Input: part model. Units: mm. Frame: model coordinates. A direction names the side the tool comes from. Give positions to 0.01 mm unless a question says otherwise; leave off trailing zeros. Loops run counter-clockwise (first coordinate to the right, second up) from the corner with the lowest first, then second, coordinate; pieces in that order, holes last. Notation, with made-up numbers: (35.25, 72) -> (80.25, 72) arc R23 cw to (80.25, 95) -> close; hole circle Ø6 at (-6, 24). An arc over 180 degrees is marked (long way). Answer as a JSON object with one key per item and string values. Group by question number.
```python
from build123d import *

# Parameters (mm, degrees)
SKETCH1_R                  = 9
SKETCH1_R_2                = 6
MAIN_DEPTH                 = 9.5
SKETCH2_W                  = 25
SKETCH2_H                  = 19
SKETCH2_R                  = 4
SKETCH2_R_2                = 1.35
BALLSUPPORTEXTRUSION_DEPTH = 5
SKETCH3_R                  = 5.15
BALLSUPPORTHOLE_DEPTH      = 4
FILLET2_R                  = 2
SKETCH5_R                  = 6
CUT_EXTRUDE2_DEPTH         = 20


with BuildPart() as part:
    # Sketch1 → Main (new body, symmetric)
    with BuildSketch(Plane.XY):
        Circle(SKETCH1_R)
        Circle(SKETCH1_R_2, mode=Mode.SUBTRACT)
    extrude(amount=MAIN_DEPTH, both=True)

    # Sketch2 → BallSupportExtrusion (add)
    with BuildSketch(Plane(origin=(0, -9, 0), x_dir=(1, 0, 0), z_dir=(0, 1, 0))):
        with Locations((12.5, 0)):
            Rectangle(SKETCH2_W, SKETCH2_H)
        with Locations((18, 0)):
            Circle(SKETCH2_R, mode=Mode.SUBTRACT)
        with Locations((18, 7)):
            Circle(SKETCH2_R_2, mode=Mode.SUBTRACT)
        with Locations((18, -7)):
            Circle(SKETCH2_R_2, mode=Mode.SUBTRACT)
    extrude(amount=BALLSUPPORTEXTRUSION_DEPTH)

    # Sketch3 → BallSupportHole (cut)
    with BuildSketch(Plane(origin=(0, -4, 0), x_dir=(1, 0, 0), z_dir=(0, 1, 0))):
        with Locations((18, 0)):
            Circle(SKETCH3_R)
    extrude(amount=-BALLSUPPORTHOLE_DEPTH, mode=Mode.SUBTRACT)

    # Fillet2
    fillet2_edges = [part.edges().sort_by_distance(p)[0] for p in [
        (8.062257748, -4, 0),
    ]]
    fillet(fillet2_edges, radius=FILLET2_R)

    # Sketch5 → Cut-Extrude2 (cut, through all)
    with BuildSketch(Plane.XY.offset(9.5)):
        Circle(SKETCH5_R)
    extrude(amount=-CUT_EXTRUDE2_DEPTH, mode=Mode.SUBTRACT)


solid = part.part
```
Q1. Ray query, probe 1 along Y at (x, z) = (0, -2.5); probe 2 along X at (y, z) = (-6.7, -7); probe 3 along Z at (x, y) = (16, -6.5). Return the intervals inside material, ascending.
Q2. Pull-direction query (X, two-part tool) for faces 4 (the face through (8, -2, 9.5)), 5 (the face through (17.824, -6.535, -8.339)), 6 (the face through (9.264, -3.26, 0.133)); classes: +X half, -X half, draft (parallel to the pull), parting line (faces both ways), or undercut.
Q3. Set-up query: faces 1 (the face through (13.91, -5.97, 3.13)), 2 (the face through (12, -9, 0)), 3 (the face through (13, -4, -2)). Return all of +Z, -Z, +X, -X, +Y, -Y with unobstructed straight access to the full face (end or side cutting, diameter ignored); none if empty.
Q4. Section D-D on x = 2. Return the cut outline in (y, z).
Q5. Pin query (flat end, axial travel): pin 1 Ø3 at (x, z) = (18, 7) entering from +Y; pin 2 Ø3 at (x, z) = (5, -1) entering from +Y; pin 3 Ø1 at (x, z) = (-4, -3) entering from -Y. Return the tip coordinate at first contact, or that it passes through.
Q6. Section A-A on y = 0. Return the cut outline in (x, z).
Q7. Section C-C on x = 18. Return the cut outline in (y, z), then the cut area to 3 significant figures.
Q8. Section B-B on z = 2.5. Return the cut outline in (x, y), then the cut area to 3 significant figures.
Numbers:
{
 "1": {"probe 1": "y = -9 to -6, 6 to 9", "probe 2": "x = -6.01 to 16.65, 19.35 to 25", "probe 3": "z = -9.5 to -4.75, 4.75 to 9.5"},
 "2": {"face 4": "draft", "face 5": "undercut", "face 6": "+X half"},
 "3": {"face 1": "+Y", "face 2": "+Z, -Z, +X, -X, -Y", "face 3": "+Z, -Z, +X, +Y"},
 "4": {"outline": "(-9, -9.5) -> (-5.66, -9.5) -> (-5.66, 9.5) -> (-9, 9.5) -> close; (5.66, -9.5) -> (8.77, -9.5) -> (8.77, 9.5) -> (5.66, 9.5) -> close"},
 "5": {"pin 1": "stops at y = -4", "pin 2": "stops at y = 8.29", "pin 3": "stops at y = -8.29"},
 "6": {"outline": "(-9, -9.5) -> (-6, -9.5) -> (-6, 9.5) -> (-9, 9.5) -> close; (6, -9.5) -> (9, -9.5) -> (9, 9.5) -> (6, 9.5) -> close"},
 "7": {"outline": "(-9, -9.5) -> (-4, -9.5) -> (-4, -8.35) -> (-9, -8.35) -> close; (-9, -5.65) -> (-4, -5.65) -> (-4, -5.15) -> (-8, -5.15) -> (-8, -4) -> (-9, -4) -> close; (-9, 4) -> (-8, 4) -> (-8, 5.15) -> (-4, 5.15) -> (-4, 5.65) -> (-9, 5.65) -> close; (-9, 8.35) -> (-4, 8.35) -> (-4, 9.5) -> (-9, 9.5) -> close", "area": "18.8 mm²"},
 "8": {"outline": "(0, -9) -> (14.88, -9) -> (14.88, -8) -> (13.5, -8) -> (13.5, -4) -> (10.82, -4) arc R2 cw to (8.85, -1.64) arc R9 ccw (long way) to start; (21.12, -9) -> (25, -9) -> (25, -4) -> (22.5, -4) -> (22.5, -8) -> (21.12, -8) -> close; hole circle Ø12 at (0, 0)", "area": "197 mm²"}
}
